Input: part model. Units: mm. Frame: model coordinates. A direction names the side the tool comes from. Round coordinates to 2 decimals unless told otherwise and drop trailing zeros. Loops run counter-clockwise (first coordinate to the right, second up) from the corner with the lowest first, then second, coordinate; pieces in that order, holes last. Notation, with made-up numbers: M 25.5,-35 L 83.5,-35 A13 cw 83.5,-10 Z; hole C 1.25,5.25 d4. An arc over 180 degrees is marked long. Return JSON: item names as keys, results as strings. Group by question number.
1) Section B-B (z = 6.5). Output: boundary loops of the cut face in (x, y), plus the area to 3 significant figures.
2) Access query for faces 5 (the face through (57, 33, 2)), 6 (the face through (62, 6, 2)), 7 (the face through (6.026, 11.352, 5.07)), 8 (the face through (15, 17, 31)). Directions: +Z, -Z, +X, -X, +Y, -Y. A direction counts if a zero-diameter tool reaches every point of the face in a straight line with its end or side. Return the directions, or none.
3) Contact query for flat-ended pins moving along their axis: P1, Ø5.5, axis at y = 40.5, z = 2, coming from the -X side; P2, Ø1.5, axis at x = 23.5, z = 3, coming from the -Y side; P3, Ø3, axis at x = 40, y = 10, coming from the +Z side; P4, Ø3, axis at y = 29.5, z = 51.5, coming from the +X side. Output: stop coordinate, or through.
4) Material intervals for line 1 (Y direction, x = 7.5, z = 3); line 2 (X direction, y = 29, z = 16); line 3 (Z direction, x = 58, y = 22), sorted ascending. Write a range as from..to.
5) Section A-A (x = 7.5). Output: boundary loops of the cut face in (y, z).
6) Mould query, pull axis Z, two halves, no side actions, for faces 1 (the face through (57.36, 40.72, 57.49)), 2 (the face through (22, 39, 5)), 3 (the face through (22.64, 24.07, 29.92)), 4 (the face through (74.408, 10.601, 5.07)). Classes: +Z half, -Z half, draft (parallel to the pull), parting line (faces both ways), or undercut.
7) Section C-C (x = 61). Output: boundary loops of the cut face in (y, z).
8) Section D-D (z = 41.5). Output: boundary loops of the cut face in (x, y), plus the area to 3 significant figures.
from build123d import *

# Parameters (mm, degrees)
SKETCH1_W           = 80
SKETCH1_H           = 45
BOSS_EXTRUDE1_DEPTH = 12
SKETCH2_W           = 15.5
SKETCH2_H           = 45
BOSS_EXTRUDE2_DEPTH = 50
SKETCH3_R           = 7.25
CUT_EXTRUDE1_DEPTH  = 50
FILLET1_R           = 15
SKETCH5_R           = 2
CUT_EXTRUDE2_DEPTH  = 50
CHAMFER1_SIZE       = 2
SKETCH6_W           = 10
SKETCH6_H           = 12
CUT_EXTRUDE3_DEPTH  = 5


with BuildPart() as part:
    # Sketch1 → Boss-Extrude1 (new body)
    with BuildSketch(Plane.XY):
        with Locations((40, 22.5)):
            Rectangle(SKETCH1_W, SKETCH1_H)
    extrude(amount=BOSS_EXTRUDE1_DEPTH)

    # Sketch2 → Boss-Extrude2 (add)
    with BuildSketch(Plane.XY.offset(12)):
        with Locations((22.75, 22.5)):
            Rectangle(SKETCH2_W, SKETCH2_H)
        with Locations((57.25, 22.5)):
            Rectangle(SKETCH2_W, SKETCH2_H)
    extrude(amount=BOSS_EXTRUDE2_DEPTH)

    # Sketch3 → Cut-Extrude1 (cut)
    with BuildSketch(Plane.ZY.offset(-15)):
        with Locations(Location((37, 22.5, 0), (0, 0, 270))):
            Circle(SKETCH3_R)
    extrude(amount=-CUT_EXTRUDE1_DEPTH, mode=Mode.SUBTRACT)

    # Fillet1
    fillet1_edges = [part.edges().sort_by_distance(p)[0] for p in [
        (22.75, 0, 62),
        (22.75, 45, 62),
        (57.25, 0, 62),
        (57.25, 45, 62),
    ]]
    fillet(fillet1_edges, radius=FILLET1_R)

    # Sketch5 → Cut-Extrude2 (cut)
    with BuildSketch(Plane.XY.offset(12)):
        with Locations((7.5, 35)):
            Circle(SKETCH5_R)
        with Locations((7.5, 10)):
            Circle(SKETCH5_R)
        with Locations((40, 35)):
            Circle(SKETCH5_R)
        with Locations((40, 10)):
            Circle(SKETCH5_R)
        with Locations((72.5, 35)):
            Circle(SKETCH5_R)
        with Locations((72.5, 10)):
            Circle(SKETCH5_R)
    extrude(amount=-CUT_EXTRUDE2_DEPTH, mode=Mode.SUBTRACT)

    # Chamfer1
    chamfer1_edges = [part.edges().sort_by_distance(p)[0] for p in [
        (5.5, 35, 12),
        (70.5, 10, 12),
        (70.5, 35, 12),
        (38, 10, 12),
        (38, 35, 12),
        (5.5, 10, 12),
    ]]
    chamfer(chamfer1_edges, length=CHAMFER1_SIZE)

    # Sketch6 → Cut-Extrude3 (cut)
    with BuildSketch(Plane(origin=(0, 0, 0), x_dir=(-1, 0, 0), z_dir=(0, 0, -1))):
        with Locations((-22, 6)):
            Rectangle(SKETCH6_W, SKETCH6_H)
        with Locations((-57, 6)):
            Rectangle(SKETCH6_W, SKETCH6_H)
        with Locations((-57, 39)):
            Rectangle(SKETCH6_W, SKETCH6_H)
        with Locations((-22, 39)):
            Rectangle(SKETCH6_W, SKETCH6_H)
    extrude(amount=-CUT_EXTRUDE3_DEPTH, mode=Mode.SUBTRACT)


solid = part.part
Returned:
{
 "1": {"outline": "M 0,0 L 80,0 L 80,45 L 0,45 Z; hole C 7.5,10 d4; hole C 7.5,35 d4; hole C 40,10 d4; hole C 40,35 d4; hole C 72.5,10 d4; hole C 72.5,35 d4", "area": "3,520 mm^2"},
 "2": {"face 5": "-Z, +Y", "face 6": "-Z, -Y", "face 7": "+Z, -Z", "face 8": "+Z, -X, +Y, -Y"},
 "3": {"P1": "stops at x = 0", "P2": "stops at y = 12", "P3": "passes through", "P4": "stops at x = 65"},
 "4": {"line 1": "y = 0..8, 12..33, 37..45", "line 2": "x = 15..30.5, 49.5..65", "line 3": "z = 0..29.77, 44.23..62"},
 "5": {"outline": "M 0,0 L 8,0 L 8,10 L 6,12 L 0,12 Z; M 12,0 L 33,0 L 33,10 L 31,12 L 14,12 L 12,10 Z; M 37,0 L 45,0 L 45,12 L 39,12 L 37,10 Z"},
 "6": {"face 1": "+Z half", "face 2": "-Z half", "face 3": "undercut", "face 4": "draft"},
 "7": {"outline": "M 0,5 L 12,5 L 12,0 L 33,0 L 33,5 L 45,5 L 45,47 A15 ccw 30,62 L 15,62 A15 ccw 0,47 Z; hole C 22.5,37 d14.5"},
 "8": {"outline": "M 15,0 L 30.5,0 L 30.5,16.82 L 15,16.82 Z; M 15,28.18 L 30.5,28.18 L 30.5,45 L 15,45 Z; M 49.5,0 L 65,0 L 65,16.82 L 49.5,16.82 Z; M 49.5,28.18 L 65,28.18 L 65,45 L 49.5,45 Z", "area": "1,040 mm^2"}
}
